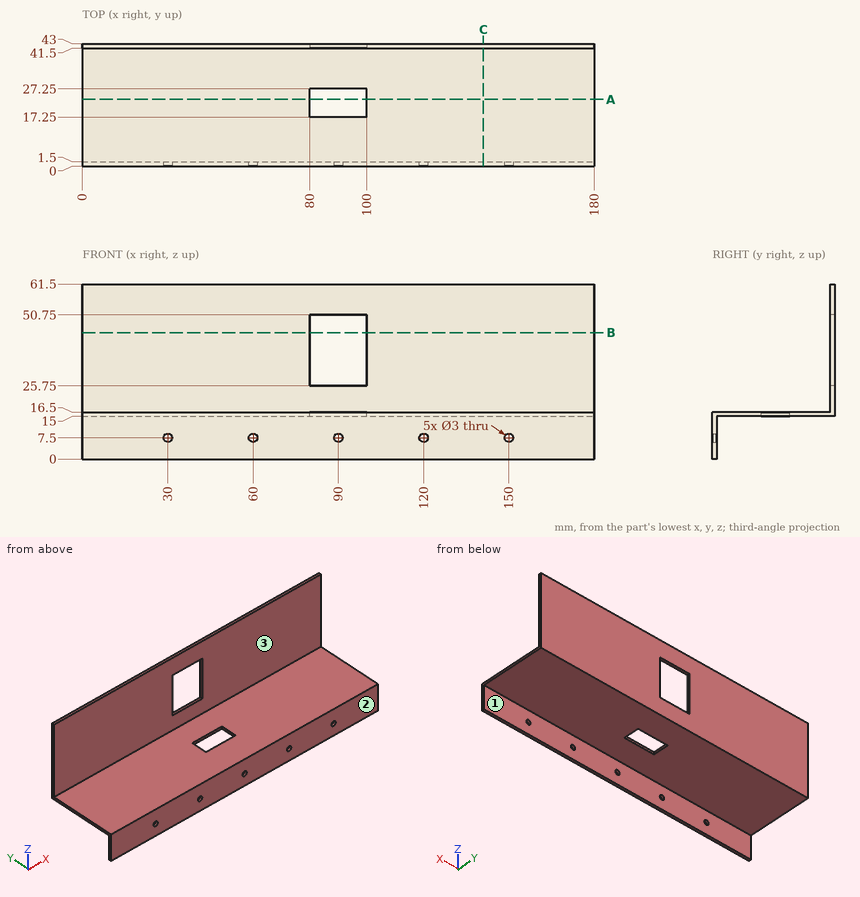
Design review of the part shown in the three views and the two pictorial views. Dimensions are in mm from the part's minimum x, y and z. A direction names the side the tool comes from. Give positions to 0.01 mm unless a question says otherwise; leave off trailing zeros. Loops run counter-clockwise (first coordinate to the right, second up) from the corner with the lowest first, then second, coordinate; pieces in that order, holes last. Notation, with made-up numbers: M 55.25,65 L 60.25,65 A18 ccw 60.25,89 Z; hole C 22.5,19.25 d6. An arc over 180 degrees is marked long. Write item = value, one per line.
Q1. Insertion check: pin 1 (1.2 mm diameter, centred on x = 91, z = 15.5, fed in from -Y); pin 2 (3.5 mm diameter, centred on x = 120, z = 7.5, fed in from +Y); pin 3 (1.2 mm diameter, centred on x = 89.5, y = 42, fed in from -Z); pin 4 (12 mm diameter, centred on x = 107.5, y = 31, fed in from +Z). Each pin has a flat end and moves straight along its axis. Give the tip position at first contact, or say it passes through.
Output values:
pin_1 = 0
pin_2 = 1.5
pin_3 = 15
pin_4 = 16.5
Q2. To check wall thickness, follow line 1 (X direction, y = 0.5, z = 7.5); line 2 (Z direction, x = 120, y = 1.05); line 3 (Y direction, x = 96, z = 18.5). State the ranges of each line that lie inside material, in increasing order. Write a range as [from, to].
Output values:
line_1 = [0, 28.5], [31.5, 58.5], [61.5, 88.5], [91.5, 118.5], [121.5, 148.5], [151.5, 180]
line_2 = [0, 6], [9, 16.5]
line_3 = [41.5, 43]
Q3. We need section C-C (x = 141). Give the boundary of the cut face in (y, z).
Output values:
outline = M 0,0 L 1.5,0 L 1.5,15 L 43,15 L 43,61.5 L 41.5,61.5 L 41.5,16.5 L 0,16.5 Z
Q4. We need section A-A (y = 23.5). Give the boundary of the cut face in (x, z).
Output values:
outline = M 0,15 L 80,15 L 80,16.5 L 0,16.5 Z; M 100,15 L 180,15 L 180,16.5 L 100,16.5 Z
Q5. We need section B-B (z = 44.5). Give the boundary of the cut face in (x, y), plus the area to 3 significant figures.
Output values:
outline = M 0,41.5 L 80,41.5 L 80,43 L 0,43 Z; M 100,41.5 L 180,41.5 L 180,43 L 100,43 Z
area = 240 mm^2
Q6. For the marked faces 1, 2 and 3, list the 3-axis set-ups (+Z, -Z, +X, -X, +Y, -Y) from which the entire face can be reached by the end or side of a thin tool; tool diameter is ignored.
Output values:
face_1 = -Z, +X, -X, +Y
face_2 = +Z, -Z, +X, -X, -Y
face_3 = +Z, +X, -X, -Y
